Input: part model. Units: mm. Frame: model coordinates. Face numbers are marked on the shaded views. A direction names the side the tool comes from. Coordinates: 2 decimals unless noted, no trailing zeros. Write each loop counter-clockwise with the first axis right and the second up, starting at its lowest first coordinate (ties: lowest second). Pieces come first, ordered by that corner, then holes. Notation, with made-up numbers: (-7, 41.25) - (29, 41.25) arc R20 cw to (29, 57.25) - close; hole circle Ø7 at (-11.5, -1.75). An arc over 180 degrees is marked (long way). Use CSV: the item, a comma, the result in double quotes.
```python
from build123d import *

# Parameters (mm, degrees)
F0_R     = 30
F0_R_2   = 14.5
F1_DEPTH = 73
F2_R     = 23.5
F2_R_2   = 14.5
F3_DEPTH = 2
F4_R     = 21
F4_R_2   = 14.5
F5_DEPTH = 5
F6_R     = 14.5
F7_DEPTH = 36
F9_DEPTH = 15.001


with BuildPart() as f1:
    # F0 (on Top) → F1 (new body)
    with BuildSketch(Plane.XY):
        Circle(F0_R)
        Circle(F0_R_2, mode=Mode.SUBTRACT)
    extrude(amount=F1_DEPTH)

    # F2 (on face) → F3 (join)
    with BuildSketch(Plane(origin=(0, 0, 0), x_dir=(1, 0, 0), z_dir=(0, 0, -1))):
        Circle(F2_R)
        Circle(F2_R_2, mode=Mode.SUBTRACT)
    extrude(amount=F3_DEPTH)

    # F4 (on face) → F5 (join)
    with BuildSketch(Plane(origin=(0, 0, -2), x_dir=(1, 0, 0), z_dir=(0, 0, -1))):
        Circle(F4_R)
        Circle(F4_R_2, mode=Mode.SUBTRACT)
    extrude(amount=F5_DEPTH)

    # F6 (on face) → F7 (cut)
    with BuildSketch(Plane.XY.offset(73)):
        with BuildLine():
            Line((15, -25.9807621135), (15, 25.9807621135))
            ThreePointArc((15, 25.9807621135), (-30, 0), (15, -25.9807621135))
        make_face()
        Circle(F6_R, mode=Mode.SUBTRACT)
        with BuildLine():
            ThreePointArc((30, 0), (28.7228132327, 8.6602540378), (25, 16.5831239518))
            Line((25, 16.5831239518), (25, -16.5831239518))
            ThreePointArc((25, -16.5831239518), (28.7228132327, -8.6602540378), (30, 0))
        make_face()
    extrude(amount=-F7_DEPTH, mode=Mode.SUBTRACT)

    # F8 (on face) → F9 (cut, through all)
    with BuildSketch(Plane(origin=(15, 0, 0), x_dir=(0, -1, 0), z_dir=(-1, 0, 0))):
        with BuildLine():
            Line((-11.5, 55), (-11.5, 40))
            ThreePointArc((-11.5, 40), (-10, 38.5), (-8.5, 40))
            Line((-8.5, 40), (-8.5, 55))
            ThreePointArc((-8.5, 55), (-10, 56.5), (-11.5, 55))
        make_face()
        with BuildLine():
            Line((8.5, 55), (8.5, 40))
            ThreePointArc((8.5, 40), (10, 38.5), (11.5, 40))
            Line((11.5, 40), (11.5, 55))
            ThreePointArc((11.5, 55), (10, 56.5), (8.5, 55))
        make_face()
        with BuildLine():
            Line((-1.5, 70), (-1.5, 57))
            ThreePointArc((-1.5, 57), (0, 55.5), (1.5, 57))
            Line((1.5, 57), (1.5, 70))
            ThreePointArc((1.5, 70), (0, 71.5), (-1.5, 70))
        make_face()
    extrude(amount=-F9_DEPTH, mode=Mode.SUBTRACT)


solid = f1.part
```
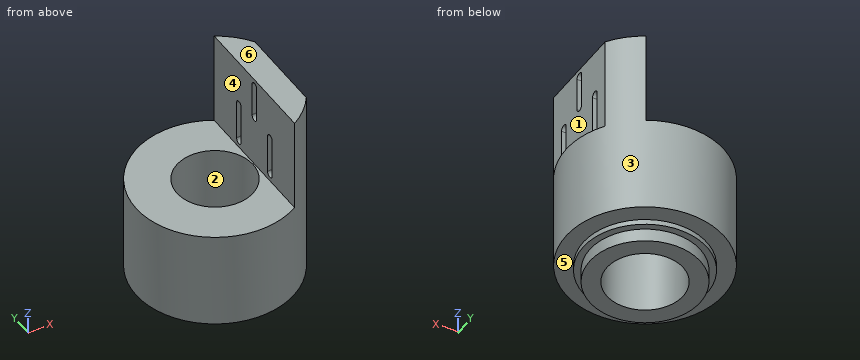
(1) Cut plane C-C on z = 65. Return loops of the section in (x, y).
Check values:
outline,"(15, -25.98) arc R30 ccw to (25, -16.58) - (25, -1.5) - (15, -1.5) - close; (15, 1.5) - (25, 1.5) - (25, 16.58) arc R30 ccw to (15, 25.98) - close"
(2) Pin query (flat end, axial travel): pin 1 Ø2 at (x, z) = (-22.5, 20.5) entering from -Y; pin 2 Ø6 at (y, z) = (10, 20) entering from -X; pin 3 Ø5 at (x, z) = (18, 47) entering from +Y. Return the tip coordinate at first contact, or that it passes through.
Check values:
pin 1,"y = -20.92"
pin 2,"x = -29.17"
pin 3,"y = 25.69"
(3) Ray query, probe 1 along X at (y, z) = (0, 23); probe 2 along Y at (x, z) = (19, 51); probe 3 along Z at (x, y) = (-7.5, 24). Return the intervals inside material, ascending. Write a range as from..to.
Check values:
probe 1,"-30..-14.5, 14.5..30"
probe 2,"-23.22..-11.5, -8.5..8.5, 11.5..23.22"
probe 3,"0..37"
(4) Reachability of the marked faces 4, 5 and 6 from +Z, -Z, +X, -X, +Y, -Y: full face, straight path, thin tool, end or side. Return the list, or none.
Check values:
face 4,"+Z, -X, +Y, -Y"
face 5,"-Z"
face 6,"+Z, +X, -X, +Y, -Y"
(5) Cut plane A-A on z = 50.5. Return loops of the section in (x, y), and give its area (3 significant figures).
Check values:
outline,"(15, -25.98) arc R30 ccw to (25, -16.58) - (25, -11.5) - (15, -11.5) - close; (15, -8.5) - (25, -8.5) - (25, 8.5) - (15, 8.5) - close; (15, 11.5) - (25, 11.5) - (25, 16.58) arc R30 ccw to (15, 25.98) - close"
area,"380 mm^2"
(6) Cut plane B-B on x = 0. Return loops of the section in (y, z), and give its area (3 significant figures).
Check values:
outline,"(-30, 0) - (-23.5, 0) - (-23.5, -2) - (-21, -2) - (-21, -7) - (-14.5, -7) - (-14.5, 37) - (-30, 37) - close; (14.5, -7) - (21, -7) - (21, -2) - (23.5, -2) - (23.5, 0) - (30, 0) - (30, 37) - (14.5, 37) - close"
area,"1,250 mm^2"
(7) Cut plane D-D on y = 4.5. Return loops of the section in (x, z), and give its area (3 significant figures).
Check values:
outline,"(-29.66, 0) - (-23.07, 0) - (-23.07, -2) - (-20.51, -2) - (-20.51, -7) - (-13.78, -7) - (-13.78, 37) - (-29.66, 37) - close; (13.78, -7) - (20.51, -7) - (20.51, -2) - (23.07, -2) - (23.07, 0) - (29.66, 0) - (29.66, 37) - (25, 37) - (25, 73) - (15, 73) - (15, 37) - (13.78, 37) - close"
area,"1,640 mm^2"
(8) Draft query along Y for the marked faces 1, 2 and 3. Return one class per face: pulls with the +Y half, pulls with the -Y half, needs draft (parallel to the pull), parting line crosses it, or undercut.
Check values:
face 1,"needs draft"
face 2,"undercut"
face 3,"parting line crosses it"
